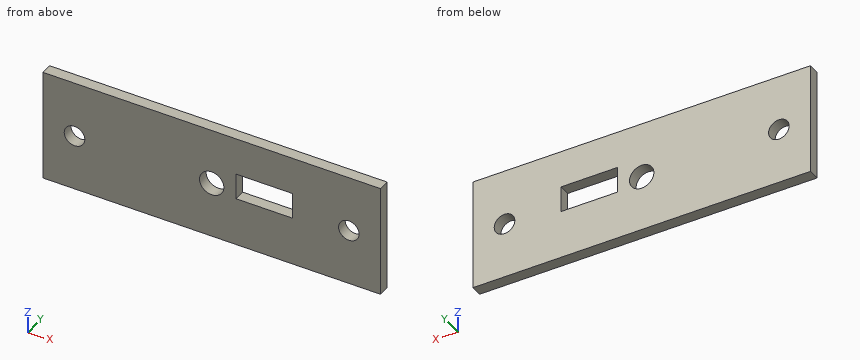
from build123d import *

# Parameters (mm, degrees)
SKETCH_1_W      = 90
SKETCH_1_H      = 30
SKETCH_1_R      = 3.25
SKETCH_1_R_2    = 2.75
SKETCH_1_W_2    = 15
SKETCH_1_H_2    = 7
EXTRUDE_1_DEPTH = 3


with BuildPart() as part:
    # Sketch 1 → Extrude 1 (new body)
    with BuildSketch(Plane(origin=(0, 0, 0), x_dir=(1, 0, 0), z_dir=(0, 1, 0))):
        Rectangle(SKETCH_1_W, SKETCH_1_H)
        with Locations(Location((0, 0, 0), (0, 0, 270))):
            Circle(SKETCH_1_R, mode=Mode.SUBTRACT)
        with Locations(Location((-36.59, 0, 0), (0, 0, 270))):
            Circle(SKETCH_1_R_2, mode=Mode.SUBTRACT)
        with Locations(Location((36.59, 0, 0), (0, 0, 270))):
            Circle(SKETCH_1_R_2, mode=Mode.SUBTRACT)
        with Locations((14, -1.5)):
            Rectangle(SKETCH_1_W_2, SKETCH_1_H_2, mode=Mode.SUBTRACT)
    extrude(amount=EXTRUDE_1_DEPTH)


solid = part.part
Input: part model. Units: mm. Frame: model coordinates. Round coordinates to 2 decimals unless told otherwise and drop trailing zeros. Order: outer loops, then holes, each group sorted by start corner. A loop starts at its lowest first (then second) coordinate and runs counter-clockwise, first axis right, second up.
1. Pin query (flat end, axial travel): P1, Ø7, axis at x = 36.59, z = 0, coming from the -Y side. Return the tip coordinate at first contact, or that it passes through.
The answers:
P1: stops at y = 0
2. Material intervals for line 1 (X direction, y = 1, z = 0); line 2 (X direction, y = 1.05, z = 4); line 3 (X direction, y = 1.3, z = 1.5), sorted ascending.
The answers:
line 1: x = -45 to -39.34, -33.84 to -3.25, 3.25 to 6.5, 21.5 to 33.84, 39.34 to 45
line 2: x = -45 to 6.5, 21.5 to 45
line 3: x = -45 to -38.89, -34.29 to -2.88, 2.88 to 6.5, 21.5 to 34.29, 38.89 to 45
3. Cut plane C-C, the plane x = 0. Output: boundary loops of the cut face in (y, z), then the cut area to 3 significant figures.
The answers:
outline: (0, -15) - (3, -15) - (3, -3.25) - (0, -3.25) - close; (0, 3.25) - (3, 3.25) - (3, 15) - (0, 15) - close
area: 70.5 mm2
4. Cut plane B-B, the plane y = 0.55. Output: boundary loops of the cut face in (x, z).
The answers:
outline: (-45, -15) - (45, -15) - (45, 15) - (-45, 15) - close; hole circle Ø5.5 at (-36.59, 0); hole circle Ø6.5 at (0, 0); hole (6.5, -2) - (21.5, -2) - (21.5, 5) - (6.5, 5) - close; hole circle Ø5.5 at (36.59, 0)
5. Cut plane A-A, the plane x = -36.59. Output: boundary loops of the cut face in (y, z), then the cut area to 3 significant figures.
The answers:
outline: (0, -15) - (3, -15) - (3, -2.75) - (0, -2.75) - close; (0, 2.75) - (3, 2.75) - (3, 15) - (0, 15) - close
area: 73.5 mm2
